Design review of the part built by this model. Coordinates are the model's own, in mm. A direction names the side the tool comes from. Give positions to 0.01 mm unless a question says otherwise; leave off trailing zeros. Loops run counter-clockwise (first coordinate to the right, second up) from the corner with the lowest first, then second, coordinate; pieces in that order, holes last. Notation, with made-up numbers: (-38, 85.5) -> (12, 85.5) arc R38 ccw to (12, 124.5) -> close; hole circle Ø8 at (13.25, -35). An arc over 180 degrees is marked (long way). Use a Markdown table: item, result. Add a question column.
1. Add section D-D (x = 33.5). State the section outline as (y, z) points, and give its area (3 significant figures).
2. Add section B-B (y = 0). State the section outline as (x, z) points.
3. For faces 1 (the flat face through (-15, 0, 0)), 2 (the flat face through (15, 0, 0)), 3 (the flat face through (-40, -10, -5)), list the 3-axis set-ups (+Z, -Z, +X, -X, +Y, -Y) from which the entire face can be reached by the end or side of a thin tool; tool diameter is ignored.
4. Add section C-C (z = 0). State the section outline as (x, y) points.
5. Add section A-A (x = 0). State the section outline as (y, z) points.
6. Draft analysis for pull direction Z (two halves, no side actions). For faces 4 (the cylindrical face through (26.914, -2.042, -9.196)), 5 (the flat face through (-1, -15, -22.5)), 6 (the cylindrical face through (-9.983, -7.655, 0.294)), state which applies: pulls with the +Z half, pulls with the -Z half, needs draft (parallel to the pull), parting line crosses it, or undercut.
7. To check wall thickness, follow line 1 (Z direction, x = -22.75, y = 0); line 2 (Y direction, x = 0, z = -3); line 3 (X direction, y = -0.5, z = 11). State the ranges of each line that lie inside material, in increasing order.
8. For pin 1 Ø21.5 at (y, z) = (0, 0) entering from +X; pin 2 Ø11.5 at (y, z) = (0, 0) entering from +X, all flat-tipped, find the tip position at first contact; note any pin that passes through.
```python
from build123d import *

# Parameters (mm, degrees)
F0_W     = 80
F0_H     = 45
F1_DEPTH = 22.5
F2_R     = 12.58
F3_DEPTH = 45.001
F4_R     = 9.42
F5_DEPTH = 25
F6_R     = 9.42
F7_DEPTH = 25
F8_SIZE  = 1.5
F9_SIZE  = 1


with BuildPart() as f1:
    # F0 (on Front) → F1 (new body, symmetric)
    with BuildSketch(Plane.XZ):
        Rectangle(F0_W, F0_H)
    extrude(amount=F1_DEPTH, both=True)

    # F2 (on face) → F3 (cut, through all)
    with BuildSketch(Plane.XY.offset(22.5)):
        Circle(F2_R)
    extrude(amount=-F3_DEPTH, mode=Mode.SUBTRACT)

    # F4 (on face) → F5 (cut)
    with BuildSketch(Plane(origin=(-40, 0, 0), x_dir=(0, -1, 0), z_dir=(-1, 0, 0))):
        Circle(F4_R)
    extrude(amount=-F5_DEPTH, mode=Mode.SUBTRACT)

    # F6 (on face) → F7 (cut)
    with BuildSketch(Plane.YZ.offset(40)):
        Circle(F6_R)
    extrude(amount=-F7_DEPTH, mode=Mode.SUBTRACT)

    # F8
    f8_edges = [f1.edges().sort_by_distance(p)[0] for p in [
        (-12.58, 0, 22.5),
        (-40, 9.42, 0),
        (-12.58, 0, -22.5),
        (40, -9.42, 0),
    ]]
    chamfer(f8_edges, length=F8_SIZE)

    # F9
    f9_edges = [f1.edges().sort_by_distance(p)[0] for p in [
        (0, -22.5, 22.5),
        (40, -22.5, 0),
        (0, -22.5, -22.5),
        (-40, -22.5, 0),
        (40, 0, 22.5),
        (0, 22.5, 22.5),
        (-40, 0, 22.5),
        (40, 0, -22.5),
        (40, 22.5, 0),
        (0, 22.5, -22.5),
        (-40, 22.5, 0),
        (-40, 0, -22.5),
    ]]
    chamfer(f9_edges, length=F9_SIZE)


solid = f1.part
```
Taken from the geometry:
| question | item | result |
|---|---|---|
| 1 | outline | (-22.5, -21.5) -> (-21.5, -22.5) -> (21.5, -22.5) -> (22.5, -21.5) -> (22.5, 21.5) -> (21.5, 22.5) -> (-21.5, 22.5) -> (-22.5, 21.5) -> close; hole circle Ø18.84 at (0, 0) |
| 1 | area | 1,740 mm^2 |
| 2 | outline | (-40, -21.5) -> (-39, -22.5) -> (-14.08, -22.5) -> (-12.58, -21) -> (-12.58, 21) -> (-14.08, 22.5) -> (-39, 22.5) -> (-40, 21.5) -> (-40, 10.92) -> (-38.5, 9.42) -> (-15, 9.42) -> (-15, -9.42) -> (-38.5, -9.42) -> (-40, -10.92) -> close; (12.58, -21) -> (14.08, -22.5) -> (39, -22.5) -> (40, -21.5) -> (40, -10.92) -> (38.5, -9.42) -> (15, -9.42) -> (15, 9.42) -> (38.5, 9.42) -> (40, 10.92) -> (40, 21.5) -> (39, 22.5) -> (14.08, 22.5) -> (12.58, 21) -> close |
| 3 | face 1 | -X |
| 3 | face 2 | +X |
| 3 | face 3 | +Z, -Z, -X, +Y, -Y |
| 4 | outline | (-40, -21.5) -> (-39, -22.5) -> (39, -22.5) -> (40, -21.5) -> (40, -10.92) -> (38.5, -9.42) -> (15, -9.42) -> (15, 9.42) -> (38.5, 9.42) -> (40, 10.92) -> (40, 21.5) -> (39, 22.5) -> (-39, 22.5) -> (-40, 21.5) -> (-40, 10.92) -> (-38.5, 9.42) -> (-15, 9.42) -> (-15, -9.42) -> (-38.5, -9.42) -> (-40, -10.92) -> close; hole circle Ø25.16 at (0, 0) |
| 5 | outline | (-22.5, -21.5) -> (-21.5, -22.5) -> (-14.08, -22.5) -> (-12.58, -21) -> (-12.58, 21) -> (-14.08, 22.5) -> (-21.5, 22.5) -> (-22.5, 21.5) -> close; (12.58, -21) -> (14.08, -22.5) -> (21.5, -22.5) -> (22.5, -21.5) -> (22.5, 21.5) -> (21.5, 22.5) -> (14.08, 22.5) -> (12.58, 21) -> close |
| 6 | face 4 | undercut |
| 6 | face 5 | pulls with the -Z half |
| 6 | face 6 | needs draft |
| 7 | line 1 | z = -22.5 to -9.42, 9.42 to 22.5 |
| 7 | line 2 | y = -22.5 to -12.58, 12.58 to 22.5 |
| 7 | line 3 | x = -40 to -12.57, 12.57 to 40 |
| 8 | pin 1 | stops at x = 39.83 |
| 8 | pin 2 | stops at x = 15 |
